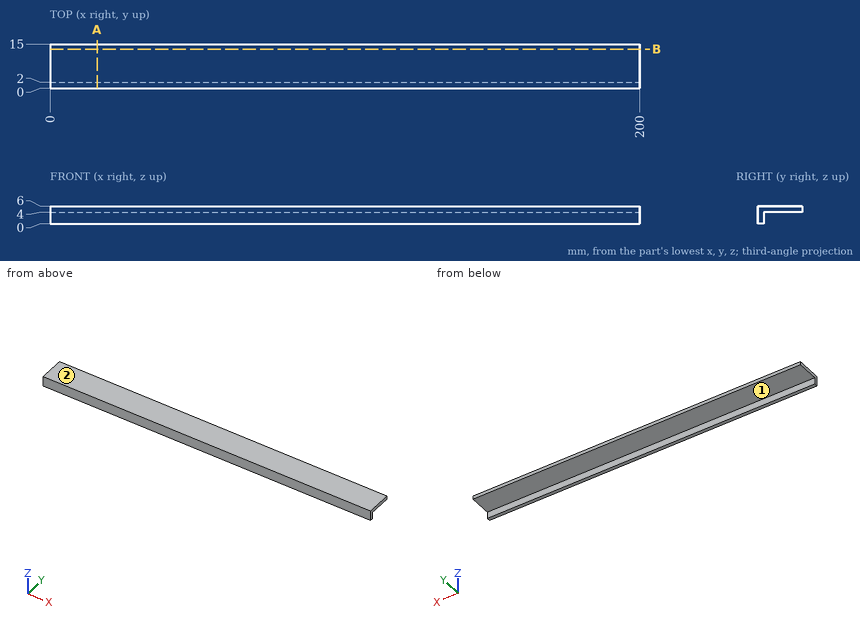
Source: three-view drawing plus pictorial views. Frame: mm from the lowest corner of the part. A direction names the side the tool comes from. Round coordinates to 2 decimals unless told otherwise and drop trailing zeros. Loops run counter-clockwise (first coordinate to the right, second up) from the corner with the lowest first, then second, coordinate; pieces in that order, holes last.
1. Section query B-B on y = 13.25. Output: boundary loops of the cut face in (x, z).
2. Contact query for flat-ended pins moving along their axis: pin 1 (3 mm diameter, centred on x = 110.5, z = 1, fed in from +Y); pin 2 (2 mm diameter, centred on y = 9, z = 5, fed in from -X); pin 3 (3 mm diameter, centred on y = 4.5, z = 1.5, fed in from -X); pin 4 (6.5 mm diameter, centred on x = 110, y = 8, fed in from -Z). Output: stop coordinate, or through.
3. Access query for the marked faces 1 and 2. Directions: +Z, -Z, +X, -X, +Y, -Y. A direction counts if a zero-diameter tool reaches every point of the face in a straight line with its end or side. Return the directions, or none.
4. Section query A-A on x = 16. Output: boundary loops of the cut face in (y, z), and give its area (3 significant figures).
5. Ray query, L1, parallel to Z at x = 125.5, y = 3; L2, parallel to Y at x = 186.5, z = 1.25. Return the intervals inside material, ascending.
Answers below:
1. outline: (0, 4) - (200, 4) - (200, 6) - (0, 6) - close
2. pin 1: stops at y = 2
2. pin 2: stops at x = 0
2. pin 3: passes through
2. pin 4: stops at z = 4
3. face 1: -Z, +X, -X, +Y
3. face 2: +Z, +X, -X, +Y, -Y
4. outline: (0, 0) - (2, 0) - (2, 4) - (15, 4) - (15, 6) - (0, 6) - close
4. area: 38.0 mm2
5. L1: z = 4 to 6
5. L2: y = 0 to 2
